Design review of the part built by this model. Coordinates are the model's own, in mm. Face numbers are marked on the shaded views. A direction names the side the tool comes from. Round coordinates to 2 decimals unless told otherwise and drop trailing zeros. Loops run counter-clockwise (first coordinate to the right, second up) from the corner with the lowest first, then second, coordinate; pieces in that order, holes last. Notation, with made-up numbers: M 26.25,73 L 42.25,73 A13 ccw 42.25,79 Z; hole C 78.25,24 d3. An arc over 180 degrees is marked long. One line per item, written item: value. Start each with the question number.
Item 1: Mouldability with a two-part tool opening along X and no side actions: class the marked faces 1, 2 and 3 as released by +X, released by -X, zero draft, split by the parting line, or undercut.
Item 2: For the marked faces 4 and 5, list the 3-axis set-ups (+Z, -Z, +X, -X, +Y, -Y) from which the entire face can be reached by the end or side of a thin tool; tool diameter is ignored.
Item 3: We need section A-A (y = 8.25). Write out the cut boundary in (x, z), then the cut area to 3 significant figures.
Item 4: For line 1 along Y through (x, z) = (15, -6.25); line 2 along X through (y, z) = (4, -5); line 3 along Z through (x, y) = (-15, 15), list the stretches that pass through material, from the lowest coordinate up.
Item 5: We need section B-B (z = 6.25). Write out the cut boundary in (x, y).
Item 6: Clearance check with flat-ended pins moving along their axes: pin 1 (2 mm diameter, centred on y = 11.684, z = -0.127, fed in from +X); pin 2 (2 mm diameter, centred on x = -5.5, z = 3.5, fed in from +Y); pin 3 (2 mm diameter, centred on x = 15.5, z = -7, fed in from +Y); pin 4 (0.8 mm diameter, centred on x = 16, y = 24.5, fed in from -Z). State where each tip first meets the part, or that it passes through.
Item 7: We need section C-C (z = 0). State how many separate pieces and enclosed holes the cut face has, then the cut area to 3 significant figures.
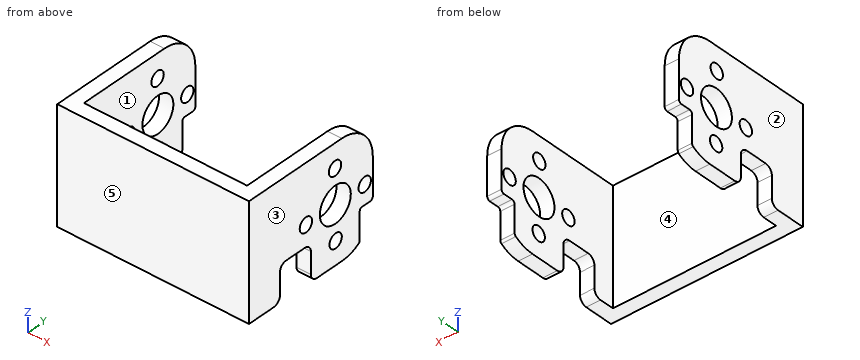
from build123d import *

# Parameters (mm, degrees)
SKETCH1_W           = 34.036
SKETCH1_H           = 20.32
BOSS_EXTRUDE1_DEPTH = 25.4
SKETCH2_W           = 28.956
SKETCH2_H           = 20.32
CUT_EXTRUDE1_DEPTH  = 22.86
SKETCH3_R           = 1.27
SKETCH3_R_2         = 3.175
CUT_EXTRUDE2_DEPTH  = 44.667320687
FILLET2_R           = 6.35
SKETCH8_W           = 6.35
SKETCH8_H           = 6.35
CUT_EXTRUDE5_DEPTH  = 44.667320687
FILLET4_R           = 1.27
SKETCH10_W          = 10.777132928
SKETCH10_H          = 6.217576688
CUT_EXTRUDE6_DEPTH  = 44.667320687
FILLET6_R           = 0.508


with BuildPart() as part:
    # Sketch1 → Boss-Extrude1 (new body)
    with BuildSketch(Plane(origin=(0, 0, 0), x_dir=(1, 0, 0), z_dir=(0, 1, 0))):
        Rectangle(SKETCH1_W, SKETCH1_H)
    extrude(amount=BOSS_EXTRUDE1_DEPTH)

    # Sketch2 → Cut-Extrude1 (cut)
    with BuildSketch(Plane(origin=(0, 25.4, 0), x_dir=(1, 0, 0), z_dir=(0, 1, 0))):
        Rectangle(SKETCH2_W, SKETCH2_H)
    extrude(amount=-CUT_EXTRUDE1_DEPTH, mode=Mode.SUBTRACT)

    # Sketch3 → Cut-Extrude2 (cut, through all)
    with BuildSketch(Plane.ZY.offset(17.018)):
        with Locations((0, 23.749)):
            Circle(SKETCH3_R)
        with Locations((-6.096, 17.78)):
            Circle(SKETCH3_R)
        with Locations((-0.127, 11.684)):
            Circle(SKETCH3_R)
        with Locations((5.969, 17.653)):
            Circle(SKETCH3_R)
        with Locations((-0.0635, 17.7165)):
            Circle(SKETCH3_R_2)
    extrude(amount=-CUT_EXTRUDE2_DEPTH, mode=Mode.SUBTRACT)

    # Fillet2
    fillet2_edges = [part.edges().sort_by_distance(p)[0] for p in [
        (-15.748, 25.4, -10.16),
        (15.748, 25.4, 10.16),
        (-15.748, 25.4, 10.16),
        (15.748, 25.4, -10.16),
    ]]
    fillet(fillet2_edges, radius=FILLET2_R)

    # Sketch8 → Cut-Extrude5 (cut, through all)
    with BuildSketch(Plane(origin=(17.018, 0, 0), x_dir=(0, 0, -1), z_dir=(1, 0, 0))):
        with Locations((6.985, 9.525)):
            Rectangle(SKETCH8_W, SKETCH8_H)
    extrude(amount=-CUT_EXTRUDE5_DEPTH, mode=Mode.SUBTRACT)

    # Fillet4
    fillet4_edges = [part.edges().sort_by_distance(p)[0] for p in [
        (15.748, 12.7, -10.16),
        (-15.748, 12.7, -10.16),
        (15.748, 6.35, -10.16),
        (-15.748, 6.35, -10.16),
        (15.748, 6.35, -3.81),
        (-15.748, 6.35, -3.81),
        (15.748, 12.7, -3.81),
        (-15.748, 12.7, -3.81),
    ]]
    fillet(fillet4_edges, radius=FILLET4_R)

    # Sketch10 → Cut-Extrude6 (cut, through all)
    with BuildSketch(Plane(origin=(17.018, 0, 0), x_dir=(0, 0, -1), z_dir=(1, 0, 0))):
        with Locations((8.813956002, 25.827034075)):
            Rectangle(SKETCH10_W, SKETCH10_H)
    extrude(amount=-CUT_EXTRUDE6_DEPTH, mode=Mode.SUBTRACT)

    # Fillet6
    fillet6_edges = [part.edges().sort_by_distance(p)[0] for p in [
        (-15.748, 22.718245731, -8.993287881),
        (15.748, 25.4, -3.425389538),
        (15.748, 22.718245731, -3.425389538),
        (-15.748, 25.4, -3.425389538),
        (-15.748, 22.718245731, -3.425389538),
        (15.748, 22.718245731, -8.993287881),
    ]]
    fillet(fillet6_edges, radius=FILLET6_R)


solid = part.part
A:
1. face 1: undercut
1. face 2: released by -X
1. face 3: released by +X
2. face 4: +Z, -Z, +Y
2. face 5: +Z, -Z, +X, -X, -Y
3. outline: M -17.02,-3.81 L -14.48,-3.81 L -14.48,10.16 L -17.02,10.16 Z; M 14.48,-3.81 L 17.02,-3.81 L 17.02,10.16 L 14.48,10.16 Z
3. area: 71.0 mm2
4. line 1: 0 to 6.35, 12.7 to 16.52, 19.04 to 22.72
4. line 2: -17.02 to -14.48, 14.48 to 17.02
4. line 3: -10.16 to -1.71, 1.58 to 10.16
5. outline: M -17.02,0 L 17.02,0 L 17.02,16.41 L 14.48,16.41 L 14.48,2.54 L -14.48,2.54 L -14.48,16.41 L -17.02,16.41 Z; M -17.02,18.89 L -14.48,18.89 L -14.48,24.91 L -17.02,24.91 Z; M 14.48,18.89 L 17.02,18.89 L 17.02,24.91 L 14.48,24.91 Z
6. pin 1: through
6. pin 2: y = 2.54
6. pin 3: y = 22.72
6. pin 4: z = -3.43
7. separate pieces: 7
7. enclosed holes: 0
7. area: 145 mm2
